Check sheet for the modelled part. Datum: model origin and axes. Units: mm. Face numbers are marked on the shaded views. Give positions to 0.01 mm unless a question says otherwise; leave off trailing zeros. Write each loop counter-clockwise with the first axis right and the second up, starting at its lowest first coordinate (ties: lowest second). Pieces come first, ordered by that corner, then holes. Notation, with made-up numbers: (44, -37.5) -> (48, -37.5) arc R33 ccw to (48, -6.5) -> close; hole circle Ø6 at (-4, -25.5). An arc over 180 degrees is marked (long way). Answer as a JSON object with one key per item and string values.
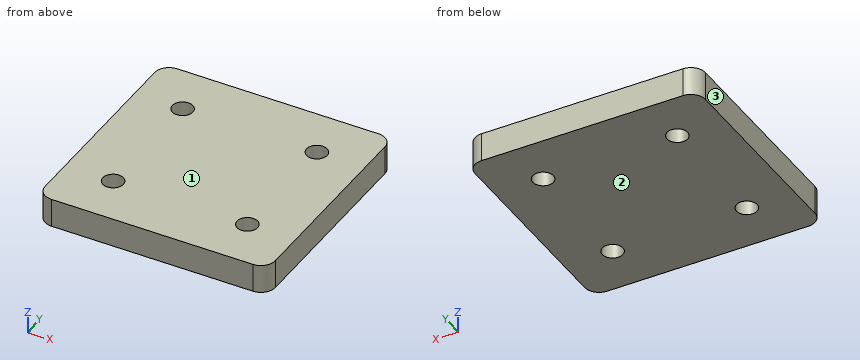
from build123d import *

# Parameters (mm, degrees)
SKETCH1_W           = 48
SKETCH1_H           = 47
SKETCH1_R           = 1.65
BOSS_EXTRUDE1_DEPTH = 6
SKETCH2_R           = 2.15
CUT_EXTRUDE1_DEPTH  = 7
FILLET1_R           = 3


with BuildPart() as part:
    # Sketch1 → Boss-Extrude1 (new body)
    with BuildSketch(Plane.XY):
        with Locations((0, -19.5)):
            Rectangle(SKETCH1_W, SKETCH1_H)
        with Locations((14, -32.5)):
            Circle(SKETCH1_R, mode=Mode.SUBTRACT)
        with Locations((-14, -32.5)):
            Circle(SKETCH1_R, mode=Mode.SUBTRACT)
        with Locations((-14, -6.5)):
            Circle(SKETCH1_R, mode=Mode.SUBTRACT)
        with Locations((14, -6.5)):
            Circle(SKETCH1_R, mode=Mode.SUBTRACT)
    extrude(amount=BOSS_EXTRUDE1_DEPTH)

    # Sketch2 → Cut-Extrude1 (cut, through all)
    with BuildSketch(Plane.XY.offset(6)):
        with Locations((-14, -6.5)):
            Circle(SKETCH2_R)
        with Locations((14, -6.5)):
            Circle(SKETCH2_R)
        with Locations((-14, -32.5)):
            Circle(SKETCH2_R)
        with Locations((14, -32.5)):
            Circle(SKETCH2_R)
    extrude(amount=-CUT_EXTRUDE1_DEPTH, mode=Mode.SUBTRACT)

    # Fillet1
    fillet1_edges = [part.edges().sort_by_distance(p)[0] for p in [
        (24, -43, 3),
        (-24, -43, 3),
        (-24, 4, 3),
        (24, 4, 3),
    ]]
    fillet(fillet1_edges, radius=FILLET1_R)


solid = part.part
1. Sectioned sample at C-C, the plane y = -32.5. Enter the section's corners in (x, z), plus the area to 3 significant figures.
Determined:
{"outline": "(-24, 0) -> (-16.15, 0) -> (-16.15, 6) -> (-24, 6) -> close; (-11.85, 0) -> (11.85, 0) -> (11.85, 6) -> (-11.85, 6) -> close; (16.15, 0) -> (24, 0) -> (24, 6) -> (16.15, 6) -> close", "area": "236 mm^2"}
2. Scan lines: L1, parallel to Y at x = -14, z = 1.5; L2, parallel to X at y = -34, z = 2.1; L3, parallel to Y at x = 15, z = 4.6. Record each from-to range of solid material in increasing order. Write a range as [from, to].
Determined:
{"L1": "[-43, -34.65], [-30.35, -8.65], [-4.35, 4]", "L2": "[-24, -15.54], [-12.46, 12.46], [15.54, 24]", "L3": "[-43, -34.4], [-30.6, -8.4], [-4.6, 4]"}
3. Mould release check, pull along Z, two halves, no side actions. Record for the marked faces 1, 2 and 3: released by +Z, released by -Z, zero draft, split by the parting line, or undercut.
Determined:
{"face 1": "released by +Z", "face 2": "released by -Z", "face 3": "zero draft"}
4. Sectioned sample at A-A, the plane x = 14. Enter the section's corners in (y, z), plus the area to 3 significant figures.
Determined:
{"outline": "(-43, 0) -> (-34.65, 0) -> (-34.65, 6) -> (-43, 6) -> close; (-30.35, 0) -> (-8.65, 0) -> (-8.65, 6) -> (-30.35, 6) -> close; (-4.35, 0) -> (4, 0) -> (4, 6) -> (-4.35, 6) -> close", "area": "230 mm^2"}
5. Sectioned sample at B-B, the plane z = 1.9. Enter the section's corners in (x, y).
Determined:
{"outline": "(-24, -40) arc R3 ccw to (-21, -43) -> (21, -43) arc R3 ccw to (24, -40) -> (24, 1) arc R3 ccw to (21, 4) -> (-21, 4) arc R3 ccw to (-24, 1) -> close; hole circle Ø4.3 at (-14, -32.5); hole circle Ø4.3 at (-14, -6.5); hole circle Ø4.3 at (14, -32.5); hole circle Ø4.3 at (14, -6.5)"}
